Autodesk Inventor part; units mm, degrees
ref_plane "YZ Plane" through (0, 0, 0) normal (1, 0, 0) x (0, 1, 0)
ref_plane "XZ Plane" through (0, 0, 0) normal (0, 1, 0) x (-1, 0, 0)
ref_plane "XY Plane" through (0, 0, 0) normal (0, 0, 1) x (1, 0, 0)
sketch "Sketch1" plane through (0, 0, 0) normal (0, 1, 0) x (-1, 0, 0)
  line L0 (0, 26.3121) -> (0, -23.4342)
  line L1 (30, -13.4342) -> (30, -3.4342)
  line L2 (25, -1.4342) -> (25, 11.5658)
  line L3 (30, -3.4342) -> (27, -3.4342)
  line L4 (28, 11.5658) -> (28, -0.4342)
  line L5 (28, -0.4342) -> (31, -0.4342)
  line L6 (33, -2.4342) -> (33, -13.4342)
  line L7 (28, 11.5658) -> (25, 11.5658)
  line L8 (27, -3.4342) -> (25, -1.4342)
  line L9 (33, -2.4342) -> (31, -0.4342)
  line L10 (30, -3.4342) -> (30, -13.4342)
  line L11 (30, -13.4342) -> (33, -13.4342)
  point P0 (0, 0)
  point P1 (25, -3.4342)
  point P2 (33, -0.4342)
  dimension "d1" = 60
  dimension "d2" = 15
  dimension "d3" = 50
  dimension "d4" = 2
  dimension "d5" = 2
  dimension "d6" = 2
  dimension "d7" = 2
revolve "Revolution1" add sketch "Sketch1" angle 360 about axis through (0, 0, 26.3121) along (0, 0, -1)
properties part number "EXTRUSSOR-COUPLING"
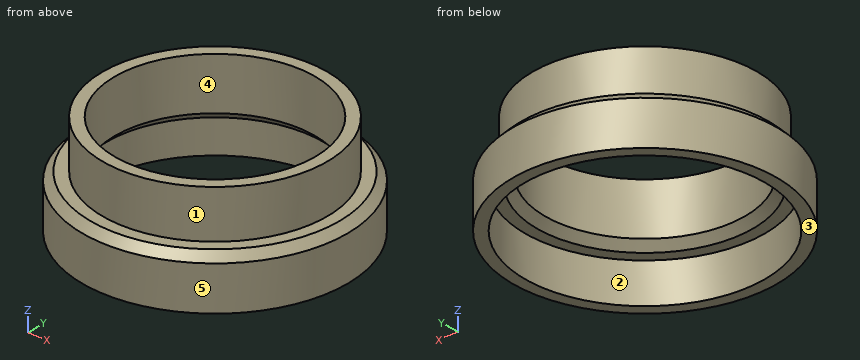
Can you work these out from the model? Positions are in its coordinate system, mm. Face numbers are marked on the shaded views. A direction names the side the tool comes from. Give positions to 0.01 mm unless a question says otherwise; leave off trailing zeros. Loops run counter-clockwise (first coordinate to the right, second up) from the corner with the lowest first, then second, coordinate; pieces in that order, holes last. Notation, with made-up numbers: M -23.5,65 L 20.5,65 A24 ccw 20.5,97 Z; hole C -17,84.25 d10. An arc over 180 degrees is marked long. One line per item, written item: value.
1) Thinking about a two-plate mould opening in Y: for the marked faces 3, 4 and 5, which applies, +Y half, -Y half, draft (parallel to the pull), parting line (faces both ways), or undercut?
Geometry check:
face 3: draft
face 4: undercut
face 5: parting line
2) Imagine slicing it at D-D on z = -8.5. Write out the boundary of the cut face in (x, y), and give its area (3 significant figures).
Geometry check:
outline: C 0,0 d66; hole C 0,0 d60
area: 594 mm²
3) Please list where these lines run through material, in increasing order: line 1 (Y direction, x = 0, z = -7); line 2 (Y direction, x = 0, z = 4.5); line 3 (X direction, y = -15.5, z = -3.5).
Geometry check:
line 1: y = -33 to -30, 30 to 33
line 2: y = -28 to -25, 25 to 28
line 3: x = -29.13 to -25.69, 25.69 to 29.13
4) Imagine slicing it at C-C on z = 7.75. Write out the boundary of the cut face in (x, y).
Geometry check:
outline: C 0,0 d56; hole C 0,0 d50
5) I'm going to push flat-ended pins straight in: pin 1 (4 mm diameter, centred on y = -7.5, z = -3, fed in from +X); pin 2 (6 mm diameter, centred on y = -9, z = -6, fed in from +X); pin 3 (1.5 mm diameter, centred on y = -23, z = 1, fed in from +X). Where does each tip first touch, or does it pass through?
Geometry check:
pin 1: stops at x = 32.54
pin 2: stops at x = 32.45
pin 3: stops at x = 17
6) On a 3-axis mill with a long thin cutter (end or side, diameter ignored), from which of +Z, -Z, +X, -X, +Y, -Y can I reach the whole of each face in a straight line? I mean the marked faces 1 and 2. Say none if no direction works.
Geometry check:
face 1: +Z
face 2: -Z
7) Imagine slicing it at A-A on x = 0. Write out the boundary of the cut face in (y, z), and give its area (3 significant figures).
Geometry check:
outline: M -33,-13.43 L -30,-13.43 L -30,-3.43 L -27,-3.43 L -25,-1.43 L -25,11.57 L -28,11.57 L -28,-0.43 L -31,-0.43 L -33,-2.43 Z; M 25,-1.43 L 27,-3.43 L 30,-3.43 L 30,-13.43 L 33,-13.43 L 33,-2.43 L 31,-0.43 L 28,-0.43 L 28,11.57 L 25,11.57 Z
area: 172 mm²
